Input: part model. Units: mm. Frame: model coordinates. A direction names the side the tool comes from. Coordinates: 2 decimals unless noted, no trailing zeros. Write each loop counter-clockwise with the first axis right and the second up, starting at its lowest first coordinate (ties: lowest second). Pieces come first, ordered by that corner, then holes. Notation, with made-up numbers: M -15.75,60 L 34.25,60 A37 ccw 34.25,96 Z; hole C -18,5 d7. An arc over 180 degrees is marked long. Use CSV: the item, a comma, the result in double quotes.
```python
from build123d import *

# Parameters (mm, degrees)
SKETCH1_W           = 38.1
SKETCH1_H           = 25.4
SKETCH1_W_2         = 31.75
SKETCH1_H_2         = 19.05
EXTRUDE_THIN1_DEPTH = 152.4
SKETCH2_R           = 3.3782
CUT_EXTRUDE1_DEPTH  = 160.130543894


with BuildPart() as part:
    # Sketch1 → Extrude-Thin1 (new body)
    with BuildSketch(Plane(origin=(0, 0, 0), x_dir=(0, 0, -1), z_dir=(1, 0, 0))):
        with Locations((19.05, 12.7)):
            Rectangle(SKETCH1_W, SKETCH1_H)
        with Locations((19.05, 12.7)):
            Rectangle(SKETCH1_W_2, SKETCH1_H_2, mode=Mode.SUBTRACT)
    extrude(amount=EXTRUDE_THIN1_DEPTH)

    # Sketch2 → Cut-Extrude1 (cut, through all)
    with BuildSketch(Plane.XY):
        with Locations((12.7, 12.7)):
            Circle(SKETCH2_R)
        with Locations((139.7, 12.7)):
            Circle(SKETCH2_R)
    extrude(amount=-CUT_EXTRUDE1_DEPTH, mode=Mode.SUBTRACT)


solid = part.part
```
1. Section B-B (x = 12.7). Return loops of the section in (y, z) (3 decimals), then the cut area to 3 significant figures.
Resolved:
outline,"M 0,-38.1 L 9.322,-38.1 L 9.322,-34.925 L 3.175,-34.925 L 3.175,-3.175 L 9.322,-3.175 L 9.322,0 L 0,0 Z; M 16.078,-38.1 L 25.4,-38.1 L 25.4,0 L 16.078,0 L 16.078,-3.175 L 22.225,-3.175 L 22.225,-34.925 L 16.078,-34.925 Z"
area,"320 mm^2"
2. Contact query for a flat-ended pin moving along its axis: pin 1 Ø4 at (x, y) = (12.7, 12.7) entering from -Z. Output: stop coordinate, or through.
Resolved:
pin 1,"passes through"
3. Access query for faces 4 (the flat face through (75, 13, -34.925)), 5 (the flat face through (75, 25.4, -19)). Directions: +Z, -Z, +X, -X, +Y, -Y. A direction counts if a zero-diameter tool reaches every point of the face in a straight line with its end or side. Return the directions, or none.
Resolved:
face 4,"+X, -X"
face 5,"+Z, -Z, +X, -X, +Y"
4. Section C-C (y = 12.7). Return loops of the section in (x, z) (3 decimals), then the cut area to 3 significant figures.
Resolved:
outline,"M 0,-38.1 L 9.322,-38.1 L 9.322,-34.925 L 0,-34.925 Z; M 0,-3.175 L 9.322,-3.175 L 9.322,0 L 0,0 Z; M 16.078,-38.1 L 136.322,-38.1 L 136.322,-34.925 L 16.078,-34.925 Z; M 16.078,-3.175 L 136.322,-3.175 L 136.322,0 L 16.078,0 Z; M 143.078,-38.1 L 152.4,-38.1 L 152.4,-34.925 L 143.078,-34.925 Z; M 143.078,-3.175 L 152.4,-3.175 L 152.4,0 L 143.078,0 Z"
area,"882 mm^2"
5. Material intervals for line 1 (Z direction, x = 79, y = 7.25) (3 decimals); line 2 (Y direction, x = 9, z = -30.5) (3 decimals); line 3 (Y direction, x = 12.7, z = -35.95), sorted ascending. Write a range as [from, to].
Resolved:
line 1,"z = [-38.1, -34.925], [-3.175, 0]"
line 2,"y = [0, 3.175], [22.225, 25.4]"
line 3,"y = [0, 9.32], [16.08, 25.4]"
6. Section A-A (z = -13.5). Return loops of the section in (x, y) (3 decimals), then the cut area to 3 significant figures.
Resolved:
outline,"M 0,0 L 152.4,0 L 152.4,3.175 L 0,3.175 Z; M 0,22.225 L 152.4,22.225 L 152.4,25.4 L 0,25.4 Z"
area,"968 mm^2"
7. Mould query, pull axis Z, two halves, no side actions, for faces 1 (the flat face through (75, 13, -38.1)), 2 (the flat face through (75, 22.225, -19)), 3 (the flat face through (75, 0, -19)). Classes: pulls with the +Z half, pulls with the -Z half, needs draft (parallel to the pull), parting line crosses it, or undercut.
Resolved:
face 1,"pulls with the -Z half"
face 2,"undercut"
face 3,"needs draft"
8. Section D-D (x = 40.5). Return loops of the section in (y, z) (3 decimals).
Resolved:
outline,"M 0,-38.1 L 25.4,-38.1 L 25.4,0 L 0,0 Z; hole M 3.175,-34.925 L 22.225,-34.925 L 22.225,-3.175 L 3.175,-3.175 Z"
